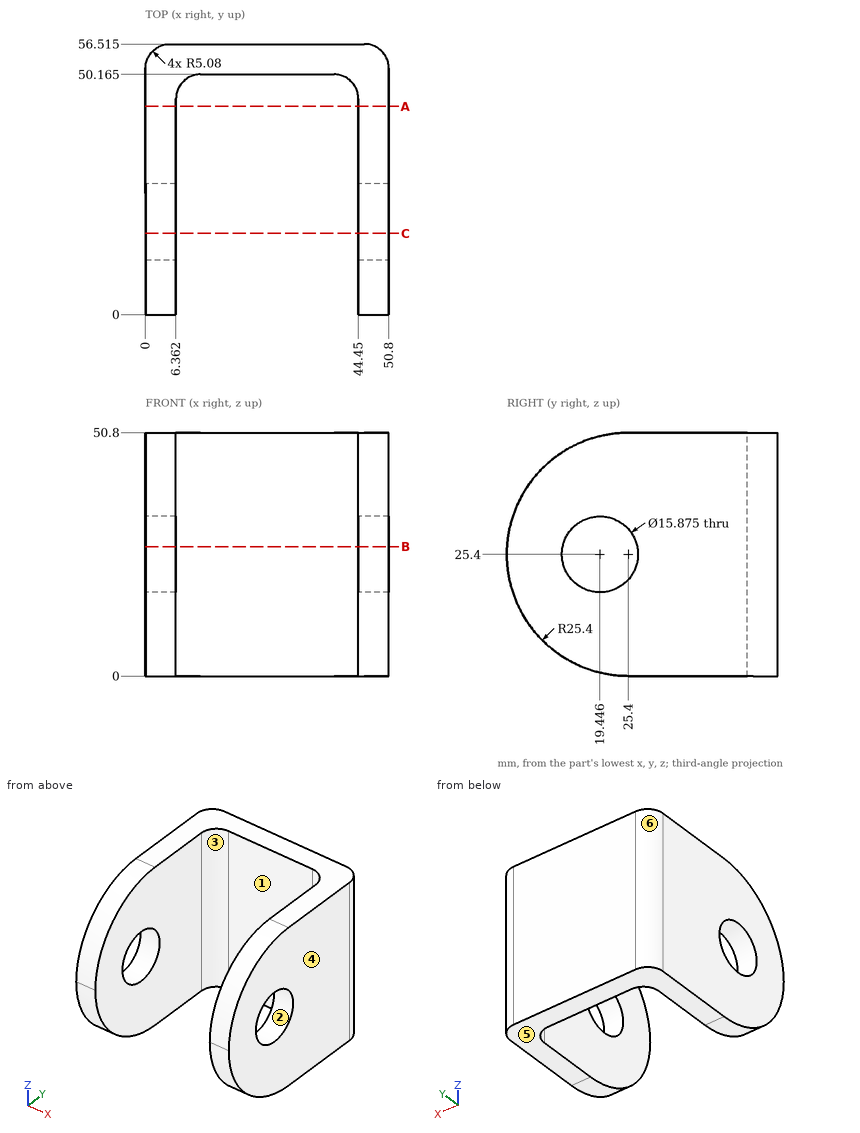
For this review, use the dimensioned drawing (mm, ordinates from the lowest corner) and the shaded views. A direction names the side the tool comes from. Give positions to 0.01 mm unless a question says otherwise; leave off trailing zeros. Order: outer loops, then holes, each group sorted by start corner. A loop starts at its lowest first (then second) coordinate and runs counter-clockwise, first axis right, second up.
1. Mouldability with a two-part tool opening along X and no side actions: class the marked faces 3, 4, 5 and 6 as +X half, -X half, draft (parallel to the pull), parting line (faces both ways), or undercut.
Solution:
face 3: undercut
face 4: +X half
face 5: draft
face 6: -X half
2. Add section B-B, the plane z = 27. State how many separate pieces and enclosed holes the cut face has, then the cut area to 3 significant figures.
Solution:
separate pieces: 3
enclosed holes: 0
area: 762 mm2
3. Add section A-A, the plane y = 43.5. State the section outline as (x, z) points, then the cut area to 3 significant figures.
Solution:
outline: (0, 0) - (6.36, 0) - (6.36, 50.8) - (0, 50.8) - close; (44.45, 0) - (50.8, 0) - (50.8, 50.8) - (44.45, 50.8) - close
area: 646 mm2
4. Add section C-C, the plane y = 17. State the section outline as (x, z) points.
Solution:
outline: (0, 1.43) - (6.36, 1.43) - (6.36, 17.85) - (0, 17.85) - close; (0, 32.95) - (6.36, 32.95) - (6.36, 49.37) - (0, 49.37) - close; (44.45, 1.43) - (50.8, 1.43) - (50.8, 17.85) - (44.45, 17.85) - close; (44.45, 32.95) - (50.8, 32.95) - (50.8, 49.37) - (44.45, 49.37) - close
5. Tool access review of the marked faces 1 and 2: name each direction out of +Z, -Z, +X, -X, +Y, -Y from which nothing blocks a thin tool from reaching the whole face with its end or side.
Solution:
face 1: +Z, -Z, -Y
face 2: +X, -X
6. For pin 1 Ø12 at (x, z) = (30, 16) entering from -Y (3 decimals), flat-tipped, find the tip position at first contact; note if it passes through.
Solution:
pin 1: stops at y = 50.165
7. To check wall thickness, follow L1, parallel to X at y = 21.5, z = 13.5; L2, parallel to Y at x = 31, z = 36.5 (1 decimal); L3, parallel to Y at x = 4, z = 25 (1 decimal). State the ranges of each line that lie inside material, in increasing order.
Solution:
L1: x = 0 to 6.36, 44.45 to 50.8
L2: y = 50.2 to 56.5
L3: y = 0 to 11.5, 27.4 to 56.4
